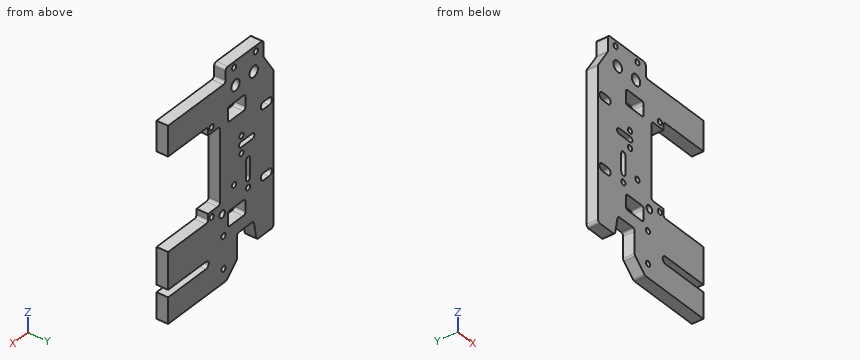
```python
from build123d import *

# Parameters (mm, degrees)
SKETCH1_R           = 1.5
SKETCH1_R_2         = 3
SKETCH1_R_3         = 2
SKETCH1_W           = 12.75
SKETCH1_H           = 8.25
BOSS_EXTRUDE1_DEPTH = 6.35
FILLET1_R           = 1.5
SKETCH3_W           = 129.678218063
SKETCH3_H           = 13.276015012
CUT_EXTRUDE1_DEPTH  = 56
SKETCH4_W           = 14.25
SKETCH4_H           = 6.35
SKETCH4_W_2         = 20.25
SKETCH4_W_3         = 16.5
BOSS_EXTRUDE2_DEPTH = 25
SKETCH5_W           = 158.83803675
SKETCH5_H           = 69.224935419
CUT_EXTRUDE2_DEPTH  = 86


with BuildPart() as part:
    # Sketch1 → Boss-Extrude1 (new body)
    with BuildSketch(Plane(origin=(0, 0, 0), x_dir=(1, 0, 0), z_dir=(0, 1, 0))):
        Polygon((0, 20), (0, 104), (12, 104), (14, 93), (26, 93), (26, 107), (33.5, 114), (62.5, 114), (70, 107), (70, 93), (82, 93), (84, 104), (96, 104), (96, 20), (89, 9), (89, 0), (62, 0), (62, 8), (34, 8), (34, 0), (7, 0), (7, 9), align=None)
        with Locations(Location((12.5, 3, 0), (0, 0, 270))):
            Circle(SKETCH1_R, mode=Mode.SUBTRACT)
        with Locations(Location((28, 3, 0), (0, 0, 270))):
            Circle(SKETCH1_R, mode=Mode.SUBTRACT)
        with Locations(Location((68, 3, 0), (0, 0, 90))):
            Circle(SKETCH1_R, mode=Mode.SUBTRACT)
        with Locations(Location((83.5, 3, 0), (0, 0, 90))):
            Circle(SKETCH1_R, mode=Mode.SUBTRACT)
        with Locations(Location((14, 13, 0), (0, 0, 270))):
            Circle(SKETCH1_R_2, mode=Mode.SUBTRACT)
        with Locations(Location((27, 13, 0), (0, 0, 270))):
            Circle(SKETCH1_R_2, mode=Mode.SUBTRACT)
        with Locations(Location((69, 13, 0), (0, 0, 90))):
            Circle(SKETCH1_R_2, mode=Mode.SUBTRACT)
        with Locations(Location((82, 13, 0), (0, 0, 90))):
            Circle(SKETCH1_R_2, mode=Mode.SUBTRACT)
        with Locations(Location((22.75, 42.455027657, 0), (0, 0, 270))):
            Circle(SKETCH1_R, mode=Mode.SUBTRACT)
        with Locations(Location((22.75, 51.751081058, 0), (0, 0, 270))):
            Circle(SKETCH1_R, mode=Mode.SUBTRACT)
        with Locations(Location((73.25, 42.455027657, 0), (0, 0, 90))):
            Circle(SKETCH1_R, mode=Mode.SUBTRACT)
        with Locations(Location((73.25, 51.751081058, 0), (0, 0, 90))):
            Circle(SKETCH1_R, mode=Mode.SUBTRACT)
        with Locations(Location((18, 72.75, 0), (0, 0, 270))):
            Circle(SKETCH1_R, mode=Mode.SUBTRACT)
        with Locations(Location((28, 65.75, 0), (0, 0, 270))):
            Circle(SKETCH1_R, mode=Mode.SUBTRACT)
        with Locations(Location((68, 65.75, 0), (0, 0, 90))):
            Circle(SKETCH1_R, mode=Mode.SUBTRACT)
        with Locations(Location((78, 72.75, 0), (0, 0, 90))):
            Circle(SKETCH1_R, mode=Mode.SUBTRACT)
        with Locations(Location((36.5, 76.75, 0), (0, 0, 270))):
            Circle(SKETCH1_R_3, mode=Mode.SUBTRACT)
        with Locations(Location((59.5, 76.75, 0), (0, 0, 90))):
            Circle(SKETCH1_R_3, mode=Mode.SUBTRACT)
        with Locations(Location((35.5, 89, 0), (0, 0, 270))):
            Circle(SKETCH1_R, mode=Mode.SUBTRACT)
        with Locations(Location((35.5, 106.5, 0), (0, 0, 270))):
            Circle(SKETCH1_R, mode=Mode.SUBTRACT)
        with Locations(Location((60.5, 89, 0), (0, 0, 90))):
            Circle(SKETCH1_R, mode=Mode.SUBTRACT)
        with Locations(Location((60.5, 106.5, 0), (0, 0, 90))):
            Circle(SKETCH1_R, mode=Mode.SUBTRACT)
        with Locations(Location((44, 26, 0), (0, 0, 270))):
            Circle(SKETCH1_R, mode=Mode.SUBTRACT)
        with Locations(Location((52, 26, 0), (0, 0, 90))):
            Circle(SKETCH1_R, mode=Mode.SUBTRACT)
        with Locations(Location((52, 74, 0), (0, 0, 270))):
            Circle(SKETCH1_R, mode=Mode.SUBTRACT)
        with Locations(Location((44, 74, 0), (0, 0, 90))):
            Circle(SKETCH1_R, mode=Mode.SUBTRACT)
        with Locations(Location((48, 97.75, 0), (0, 0, 270))):
            Circle(SKETCH1_R_3, mode=Mode.SUBTRACT)
        with Locations((69.875, 25.875)):
            Rectangle(SKETCH1_W, SKETCH1_H, mode=Mode.SUBTRACT)
        with Locations((26.125, 25.875)):
            Rectangle(SKETCH1_W, SKETCH1_H, mode=Mode.SUBTRACT)
        with Locations((69.875, 81.875)):
            Rectangle(SKETCH1_W, SKETCH1_H, mode=Mode.SUBTRACT)
        with Locations((26.125, 81.875)):
            Rectangle(SKETCH1_W, SKETCH1_H, mode=Mode.SUBTRACT)
        with BuildLine():
            Line((3, 75), (7, 75))
            ThreePointArc((7, 75), (9, 73), (7, 71))
            Line((7, 71), (3, 71))
            ThreePointArc((3, 71), (1, 73), (3, 75))
        make_face(mode=Mode.SUBTRACT)
        with BuildLine():
            Line((93, 75), (89, 75))
            ThreePointArc((89, 75), (87, 73), (89, 71))
            Line((89, 71), (93, 71))
            ThreePointArc((93, 71), (95, 73), (93, 75))
        make_face(mode=Mode.SUBTRACT)
        with BuildLine():
            Line((93, 37), (89, 37))
            ThreePointArc((89, 37), (87, 35), (89, 33))
            Line((89, 33), (93, 33))
            ThreePointArc((93, 33), (95, 35), (93, 37))
        make_face(mode=Mode.SUBTRACT)
        with BuildLine():
            Line((3, 33), (7, 33))
            ThreePointArc((7, 33), (9, 35), (7, 37))
            Line((7, 37), (3, 37))
            ThreePointArc((3, 37), (1, 35), (3, 33))
        make_face(mode=Mode.SUBTRACT)
        with BuildLine():
            Line((15, 48.525154469), (23, 48.525154469))
            ThreePointArc((23, 48.525154469), (24.5, 47.025154469), (23, 45.525154469))
            Line((23, 45.525154469), (15, 45.525154469))
            ThreePointArc((15, 45.525154469), (13.5, 47.025154469), (15, 48.525154469))
        make_face(mode=Mode.SUBTRACT)
        with BuildLine():
            Line((81, 48.525154469), (73, 48.525154469))
            ThreePointArc((73, 48.525154469), (71.5, 47.025154469), (73, 45.525154469))
            Line((73, 45.525154469), (81, 45.525154469))
            ThreePointArc((81, 45.525154469), (82.5, 47.025154469), (81, 48.525154469))
        make_face(mode=Mode.SUBTRACT)
        with BuildLine():
            Line((16.5, 67.75), (16.5, 57.75))
            ThreePointArc((16.5, 57.75), (18, 56.25), (19.5, 57.75))
            Line((19.5, 57.75), (19.5, 67.75))
            ThreePointArc((19.5, 67.75), (18, 69.25), (16.5, 67.75))
        make_face(mode=Mode.SUBTRACT)
        with BuildLine():
            Line((76.5, 67.75), (76.5, 57.75))
            ThreePointArc((76.5, 57.75), (78, 56.25), (79.5, 57.75))
            Line((79.5, 57.75), (79.5, 67.75))
            ThreePointArc((79.5, 67.75), (78, 69.25), (76.5, 67.75))
        make_face(mode=Mode.SUBTRACT)
        with BuildLine():
            Line((46.5, 29), (38, 29))
            Line((38, 29), (38, 71))
            Line((38, 71), (46.5, 71))
            Line((46.5, 71), (46.5, 74))
            ThreePointArc((46.5, 74), (48, 75.5), (49.5, 74))
            Line((49.5, 74), (49.5, 71))
            Line((49.5, 71), (58, 71))
            Line((58, 71), (58, 29))
            Line((58, 29), (49.5, 29))
            Line((49.5, 29), (49.5, 26))
            ThreePointArc((49.5, 26), (48, 24.5), (46.5, 26))
            Line((46.5, 26), (46.5, 29))
        make_face(mode=Mode.SUBTRACT)
    extrude(amount=BOSS_EXTRUDE1_DEPTH)

    # Fillet1
    fillet1_edges = [part.edges().sort_by_distance(p)[0] for p in [
        (19.75, 3.175, -30),
        (19.75, 3.175, -21.75),
        (32.5, 3.175, -21.75),
        (32.5, 3.175, -30),
        (63.5, 3.175, -77.75),
        (76.25, 3.175, -77.75),
        (76.25, 3.175, -86),
        (63.5, 3.175, -86),
        (19.75, 3.175, -86),
        (19.75, 3.175, -77.75),
        (32.5, 3.175, -77.75),
        (32.5, 3.175, -86),
        (58, 3.175, -29),
        (58, 3.175, -71),
        (38, 3.175, -71),
        (38, 3.175, -29),
        (62, 3.175, -8),
        (34, 3.175, -8),
        (34, 3.175, 0),
        (7, 3.175, 0),
        (7, 3.175, -9),
        (0, 3.175, -20),
        (0, 3.175, -104),
        (12, 3.175, -104),
        (14, 3.175, -93),
        (26, 3.175, -93),
        (26, 3.175, -107),
        (33.5, 3.175, -114),
        (62.5, 3.175, -114),
        (70, 3.175, -107),
        (70, 3.175, -93),
        (82, 3.175, -93),
        (84, 3.175, -104),
        (96, 3.175, -104),
        (96, 3.175, -20),
        (89, 3.175, -9),
        (89, 3.175, 0),
        (62, 3.175, 0),
        (76.25, 3.175, -21.75),
        (76.25, 3.175, -30),
        (63.5, 3.175, -30),
        (63.5, 3.175, -21.75),
    ]]
    fillet(fillet1_edges, radius=FILLET1_R)

    # Sketch3 → Cut-Extrude1 (cut)
    with BuildSketch(Plane(origin=(48, 0, 0), x_dir=(0, 0, -1), z_dir=(1, 0, 0))):
        with Locations((58.42243018, 0.940732076)):
            Rectangle(SKETCH3_W, SKETCH3_H)
    extrude(amount=CUT_EXTRUDE1_DEPTH, mode=Mode.SUBTRACT)

    # Sketch4 → Boss-Extrude2 (add)
    with BuildSketch(Plane(origin=(48, 0, 0), x_dir=(0, 0, -1), z_dir=(1, 0, 0))):
        with Locations((106.875, 3.175)):
            Rectangle(SKETCH4_W, SKETCH4_H)
        with Locations((85.625, 3.175)):
            Rectangle(SKETCH4_W_2, SKETCH4_H)
        with Locations((16.25, 3.175)):
            Rectangle(SKETCH4_W_3, SKETCH4_H)
    extrude(amount=BOSS_EXTRUDE2_DEPTH)

    # Mirror1: part across plane


with BuildPart() as part_1:
    add(part.part)
    add(part.part.mirror(Plane(origin=(73, 0, 0), x_dir=(0, 0, 1), z_dir=(1, 0, 0))))

    # Sketch5 → Cut-Extrude2 (cut)
    with BuildSketch(Plane(origin=(75, 0, 0), x_dir=(0, 0, -1), z_dir=(1, 0, 0))):
        with Locations((54.73207584, 3.767679241)):
            Rectangle(SKETCH5_W, SKETCH5_H)
    extrude(amount=CUT_EXTRUDE2_DEPTH, mode=Mode.SUBTRACT)


solid = part_1.part
```
Could you check a few things on this model? Use its own coordinates, in mm. Round coordinates to 2 decimals unless told otherwise and drop trailing zeros. Loops run counter-clockwise (first coordinate to the right, second up) from the corner with the lowest first, then second, coordinate; pieces in that order, holes last. Notation, with made-up numbers: M 58.25,68.25 L 67.25,68.25 A14 cw 67.25,74.25 Z; hole C 36,66 d3. An arc over 180 degrees is marked long. Put each result on its own line as item: value.
Q1. Imagine slicing it at A-A (x = 69). Write out the boundary of the cut face in (y, z).
Check result:
outline: M 0,-114 L 6.35,-114 L 6.35,-99.75 L 0,-99.75 Z; M 0,-95.75 L 6.35,-95.75 L 6.35,-75.5 L 0,-75.5 Z; M 0,-24.5 L 6.35,-24.5 L 6.35,-8 L 0,-8 Z
Q2. I need wall thicknesses on probe 1 along Z at (x, y) = (51, 4); probe 2 along X at (y, z) = (3.25, -65.75); probe 3 along X at (y, z) = (2.25, -3). Which ranges of each line are inside material? Lowest first, please.
Check result:
probe 1: -114 to -99.75, -95.75 to -75.5, -24.5 to -8
probe 2: 0 to 16.5, 19.5 to 26.5, 29.5 to 38
probe 3: 7 to 11, 14 to 26.5, 29.5 to 34
Q3. For pin 1 (2.5 mm diameter, centred on x = 28, z = -3, fed in from +Y); pin 2 (1.5 mm diameter, centred on y = 3, z = -32, fed in from +X); pin 3 (1 mm diameter, centred on x = 42.5, y = 4.5, fed in from +Z); pin 4 (1.2 mm diameter, centred on x = 4, y = 4, fed in from +Z), each with a flat end and sliding along its axis, tell me the tip position at first contact or that it passes through.
Check result:
pin 1: through
pin 2: x = 38
pin 3: z = -8
pin 4: z = -12.77
Q4. Imagine slicing it at B-B (z = -3). Write out the boundary of the cut face in (x, y), then the cut area to 3 significant figures.
Check result:
outline: M 7,0 L 11,0 L 11,6.35 L 7,6.35 Z; M 14,0 L 26.5,0 L 26.5,6.35 L 14,6.35 Z; M 29.5,0 L 34,0 L 34,6.35 L 29.5,6.35 Z
area: 133 mm2
Q5. Imagine slicing it at C-C (x = 44). Write out the boundary of the cut face in (y, z).
Check result:
outline: M 0,-114 L 6.35,-114 L 6.35,-75.5 L 0,-75.5 Z; M 0,-72.5 L 6.35,-72.5 L 6.35,-71 L 0,-71 Z; M 0,-29 L 6.35,-29 L 6.35,-27.5 L 0,-27.5 Z; M 0,-24.5 L 6.35,-24.5 L 6.35,-8 L 0,-8 Z
Q6. Imagine slicing it at D-D (z = -35). Write out the boundary of the cut face in (x, y), then the cut area to 4 significant figures.
Check result:
outline: M 0,0 L 1,0 L 1,6.35 L 0,6.35 Z; M 9,0 L 38,0 L 38,6.35 L 9,6.35 Z
area: 190.5 mm2
